from build123d import *

# Parameters (mm, degrees)
SKETCH2_W           = 45
SKETCH2_H           = 25
BOSS_EXTRUDE1_DEPTH = 2
SKETCH3_W           = 45
SKETCH3_H           = 25
SKETCH3_W_2         = 37
SKETCH3_H_2         = 17
BOSS_EXTRUDE2_DEPTH = 35
BOSS_EXTRUDE2_TAPER = 6


with BuildPart() as part:
    # Sketch2 → Boss-Extrude1 (new body)
    with BuildSketch(Plane(origin=(0, 0, 0), x_dir=(1, 0, 0), z_dir=(0, 1, 0))):
        Rectangle(SKETCH2_W, SKETCH2_H)
    extrude(amount=BOSS_EXTRUDE1_DEPTH)

    # Sketch3 → Boss-Extrude2 (add)
    with BuildSketch(Plane(origin=(0, 2, 0), x_dir=(1, 0, 0), z_dir=(0, 1, 0))):
        Rectangle(SKETCH3_W, SKETCH3_H)
        Rectangle(SKETCH3_W_2, SKETCH3_H_2, mode=Mode.SUBTRACT)
    extrude(amount=BOSS_EXTRUDE2_DEPTH, taper=BOSS_EXTRUDE2_TAPER)


solid = part.part
Could you check a few things on this model? Use its own coordinates, in mm. Round coordinates to 2 decimals unless told otherwise and drop trailing zeros.
(1) If we mould it in two halves opening along Z, with no side actions, what happens to faces 1 (the flat face through (0, 1, -12.5)), 2 (the flat face through (0, 2, 0)), 3 (the flat face through (0, 1, 12.5)), 4 (the flat face through (22.5, 1, 0))? For each: released by +Z, released by -Z, zero draft, split by the parting line, or undercut.
Response values:
face 1: released by -Z
face 2: undercut
face 3: released by +Z
face 4: zero draft
(2) I'm going to push flat-ended pins straight in: pin 1 (1 mm diameter, centred on x = 8, z = 8.5, fed in from -Y); pin 2 (1.5 mm diameter, centred on x = -17.5, y = 13, fed in from -Z); pin 3 (3 mm diameter, centred on y = 16.5, z = 5, fed in from -X); pin 4 (8 mm diameter, centred on y = 12, z = -2, fed in from -X). Where does each tip first touch, or does it pass through?
Response values:
pin 1: stops at y = 0
pin 2: stops at z = -11.42
pin 3: stops at x = -21.13
pin 4: stops at x = -21.87
(3) Please list where these lines run through material, in increasing order: line 1 along Z through (x, y) = (-10, 15); line 2 along Y through (x, z) = (11.5, -6.5); line 3 along Z through (x, y) = (7, 7.25).
Response values:
line 1: z = -11.13 to -9.87, 9.87 to 11.13
line 2: y = 0 to 2
line 3: z = -11.95 to -9.05, 9.05 to 11.95
